Autodesk Fusion 360 part; units mm, degrees
sketch "Sketch1" plane through (0, 0, 0) normal (0, 0, 1) x (1, 0, 0)
  line L0 (0, 0) -> (60, 0)
  line L1 (60, 0) -> (60, 50)
  line L2 (60, 50) -> (0, 50)
  line L3 (0, 50) -> (0, 0)
  line L4 (0, 50) -> (5, 50)
  line L5 (5, 50) -> (5, 47.5)
  line L6 (5, 47.5) -> (0, 47.5)
  line L7 (0, 47.5) -> (0, 50)
  line L8 (0, 0) -> (5, 0)
  line L9 (5, 0) -> (5, 2.5)
  line L10 (5, 2.5) -> (0, 2.5)
  line L11 (0, 2.5) -> (0, 0)
  circle A0 centre (5, 2.5) radius 1.5
  circle A1 centre (5, 47.5) radius 1.5
  line L12 (5, 47.5) -> (35, 47.5)
  line L13 (5, 2.5) -> (35, 2.5)
  line L14 (5, 50) -> (5, 40)
  line L15 (5, 0) -> (5, 10)
  line L16 (5, 40) -> (50, 40)
  line L17 (5, 10) -> (50, 10)
  line L18 (60, 50) -> (60, 45)
  line L19 (60, 45) -> (45, 45)
  circle A2 centre (45, 45) radius 1.25
  line L20 (60, 0) -> (60, 5)
  line L21 (60, 5) -> (45, 5)
  circle A3 centre (45, 5) radius 1.25
  line L22 (60, 0) -> (60, 25)
  line L23 (60, 25) -> (45, 25)
  circle A4 centre (45, 25) radius 6.25
  circle A5 centre (50, 40) radius 1.5
  circle A6 centre (5, 10) radius 1.5
  circle A7 centre (50, 10) radius 1.5
  circle A8 centre (35, 47.5) radius 1.5
  circle A9 centre (35, 2.5) radius 1.5
  dimension "d1" = 60
  dimension "d2" = 50
  dimension "d3" = 5
  dimension "d4" = 2.5
  dimension "d5" = 5
  dimension "d6" = 2.5
  dimension "d7" = 3
  dimension "d8" = 3
  dimension "d9" = 30
  dimension "d10" = 30
  dimension "d11" = 10
  dimension "d12" = 10
  dimension "d13" = 45
  dimension "d14" = 45
  dimension "d15" = 15
  dimension "d16" = 2.5
  dimension "d17" = 5
  dimension "d18" = 15
  dimension "d19" = 2.5
  dimension "d20" = 15
  dimension "d21" = 12.5
  dimension "d22" = 3
  dimension "d23" = 3
  dimension "d24" = 3
  dimension "d25" = 3
  dimension "d26" = 3
extrude "Extrude1" add sketch "Sketch1" along normal blind 5 contours L0 L3 L8 L9 L10 L11 A0 L15 | L0 L1 L2 L3 L5 L6 L9 L10 A0 A1 L14 L15 L18 L20 L22 | L2 L3 L4 L5 L6 L7 A1 L14
sketch "Sketch2" plane through (0, 0, 5) normal (0, 0, 1) x (1, 0, 0)
  circle A0 centre (5, 2.5) radius 1.5
  circle A1 centre (5, 10) radius 1.5
  circle A2 centre (35, 2.5) radius 1.5
  circle A3 centre (45, 45) radius 1.25
  circle A4 centre (35, 47.5) radius 1.5
  circle A5 centre (50, 40) radius 1.5
  circle A6 centre (50, 10) radius 1.5
  circle A7 centre (45, 5) radius 1.25
  circle A8 centre (45, 25) radius 6.25
  circle A9 centre (5, 47.5) radius 1.5
  line L0 (0, 50) -> (0, 0)
  line L1 (0, 0) -> (60, 0)
  line L2 (60, 0) -> (60, 50)
  line L3 (60, 50) -> (0, 50)
  line L4 (50, 40) -> (5, 40)
  circle A10 centre (5, 40) radius 1.5
  dimension "d29" = 45
  dimension "d30" = 3
extrude "Extrude2" cut sketch "Sketch2" against normal blind 5 contours A10
sketch "Sketch3" plane through (0, 0, 0) normal (0, 0, -1) x (-1, 0, 0)
  circle A0 centre (-5, 40) radius 1.5
  circle A1 centre (-5, 2.5) radius 1.5
  circle A2 centre (-5, 10) radius 1.5
  circle A3 centre (-35, 2.5) radius 1.5
  circle A4 centre (-45, 45) radius 1.25
  circle A5 centre (-35, 47.5) radius 1.5
  circle A6 centre (-50, 40) radius 1.5
  circle A7 centre (-50, 10) radius 1.5
  circle A8 centre (-45, 5) radius 1.25
  circle A9 centre (-45, 25) radius 6.25
  circle A10 centre (-5, 47.5) radius 1.5
  line L0 (0, 0) -> (0, 50)
  line L1 (0, 50) -> (-60, 50)
  line L2 (-60, 50) -> (-60, 0)
  line L3 (-60, 0) -> (0, 0)
  line L4 (0, 0) -> (-10, 0)
  line L5 (-10, 0) -> (-14, 0)
  line L6 (-14, 0) -> (-14, 30)
  line L7 (-14, 30) -> (-10, 30)
  line L8 (-10, 30) -> (-10, 0)
  dimension "d33" = 10
  dimension "d34" = 4
  dimension "d35" = 30
extrude "Extrude3" add sketch "Sketch3" along normal blind 20 contours L3 L5 L6 L7 L8
sketch "Sketch4" plane through (0, 0, -20) normal (0, 0, -1) x (-1, 0, 0)
  line L0 (-10, 30) -> (-14, 30)
  line L1 (-14, 30) -> (-14, 0)
  line L2 (-14, 0) -> (-10, 0)
  line L3 (-10, 0) -> (-10, 30)
  line L4 (-14, 30) -> (-10, 30)
  line L5 (-10, 30) -> (-10, 26.5)
  line L6 (-10, 26.5) -> (-14, 26.5)
  line L7 (-14, 26.5) -> (-14, 30)
  line L8 (-10, 0) -> (-14, 0)
  line L9 (-14, 0) -> (-14, 3.5)
  line L10 (-14, 3.5) -> (-10, 3.5)
  line L11 (-10, 3.5) -> (-10, 0)
  dimension "d38" = 3.5
  dimension "d39" = 3.5
extrude "Extrude4" add sketch "Sketch4" along normal blind 10 contours L0 L1 L3 L4 L5 L6 L7 | L1 L2 L3 L8 L9 L10 L11
sketch "Sketch5" plane through (10, 0, 0) normal (-1, 0, 0) x (0, 0, 1)
  line L0 (0, 0) -> (0, 30)
  line L1 (0, 30) -> (-30, 30)
  line L2 (-30, 30) -> (-30, 26.5)
  line L3 (-30, 26.5) -> (-20, 26.5)
  line L4 (-20, 26.5) -> (-20, 3.5)
  line L5 (-20, 3.5) -> (-30, 3.5)
  line L6 (-30, 3.5) -> (-30, 0)
  line L7 (-30, 0) -> (0, 0)
  line L8 (-30, 30) -> (-30, 28.25)
  line L9 (-30, 28.25) -> (-25, 28.25)
  line L10 (-30, 0) -> (-30, 1.75)
  line L11 (-30, 1.75) -> (-25, 1.75)
  circle A0 centre (-25, 28.25) radius 1
  circle A1 centre (-25, 1.75) radius 1
  dimension "d42" = 5
  dimension "d43" = 2
  dimension "d44" = 2
extrude "Extrude5" cut sketch "Sketch5" against normal blind 4 contours A0 | A1
sketch "Sketch6" plane through (0, 0, 0) normal (0, 0, -1) x (-1, 0, 0)
  line L0 (-14, 0) -> (-14, 30)
  line L1 (-14, 30) -> (-10, 30)
  line L2 (-10, 30) -> (-10, 0)
  line L3 (-10, 0) -> (0, 0)
  line L4 (0, 0) -> (0, 50)
  line L5 (0, 50) -> (-60, 50)
  line L6 (-60, 50) -> (-60, 0)
  line L7 (-60, 0) -> (-14, 0)
  circle A0 centre (-5, 47.5) radius 1.5
  circle A1 centre (-45, 25) radius 6.25
  circle A2 centre (-45, 5) radius 1.25
  circle A3 centre (-50, 10) radius 1.5
  circle A4 centre (-50, 40) radius 1.5
  circle A5 centre (-35, 47.5) radius 1.5
  circle A6 centre (-45, 45) radius 1.25
  circle A7 centre (-35, 2.5) radius 1.5
  circle A8 centre (-5, 10) radius 1.5
  circle A9 centre (-5, 2.5) radius 1.5
  circle A10 centre (-5, 40) radius 1.5
  line L8 (-10, 0) -> (-10, 5)
  line L9 (-10, 30) -> (-10, 25)
  line L10 (-10, 5) -> (0, 5)
  line L11 (0, 5) -> (0, 8)
  line L12 (0, 8) -> (-10, 8)
  line L13 (-10, 8) -> (-10, 5)
  line L14 (-10, 25) -> (0, 25)
  line L15 (0, 25) -> (0, 22)
  line L16 (0, 22) -> (-10, 22)
  line L17 (-10, 22) -> (-10, 25)
  dimension "d47" = 5
  dimension "d48" = 3
extrude "Extrude6" add sketch "Sketch6" along normal blind 20 contours L2 L4 L14 L15 L16 L17 | L2 L4 L10 L11 L12 L13
chamfer "Chamfer1" distance 10 distance2 20 2 edges at (0, 23.5, -20) (0, 6.5, -20) measured on face at (12.6667, 12.6667, -20) measured on face at (12.6667, 12.6667, -20)
extrude "Extrude7" add 1 faces at (12.6667, 30, -10) along direction (0, 1, 0) blind 3
extrude "Extrude8" add 1 faces at (24.6667, 0, 3.3333) along direction (0, -1, 0) blind 3
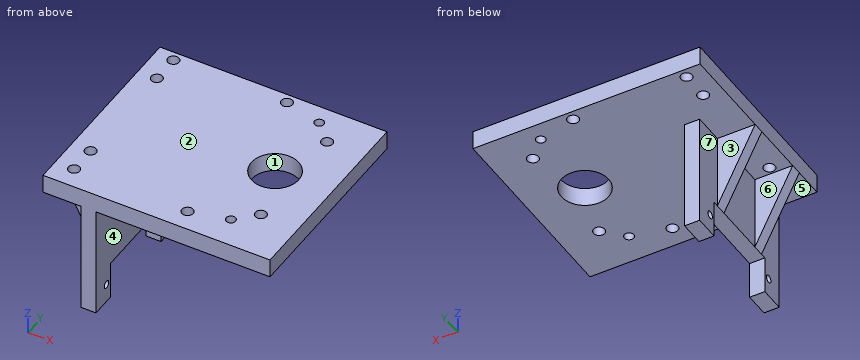
The listing builds one solid part. Answer for the finished solid, in the listing's coordinates (mm). Face numbers are marked on the shaded views. A direction names the side the tool comes from. Give positions to 0.01 mm unless a question says otherwise; leave off trailing zeros. Order: outer loops, then holes, each group sorted by start corner. A loop starts at its lowest first (then second) coordinate and runs counter-clockwise, first axis right, second up. Notation, with made-up numbers: (-34, 52.5) -> (0, 52.5) arc R11 ccw to (0, 73.5) -> close; hole circle Ø11 at (43, 74). An arc over 180 degrees is marked (long way). Answer as a JSON object with one key per item and string values. Group by question number.
Item 1: The part is cut by section D-D on x = 45. Write down the section's boundary in (y, z).
Item 2: The part is cut by section B-B on x = 35. Write down the section's boundary in (y, z).
Item 3: The part is cut by section C-C on z = -25. Write down the section's boundary in (x, y).
Item 4: A tool of negligible diameter and unlimited length cuts with its end or side. For the marked faces 4, 5, 6 and 7, from which of +Z, -Z, +X, -X, +Y, -Y can it reach the whole face along a straight path? Write none if from no direction.
Item 5: The part is cut by section A-A on y = 45. Write down the section's boundary in (x, z), and give its area (4 significant figures).
Item 6: Determine the mould class of the marked faces 1, 2 and 3 for opening direction Y: pulls with the +Y half, pulls with the -Y half, needs draft (parallel to the pull), parting line crosses it, or undercut.
Item 7: Consider L1, parallel to X at y = 40, z = 3; L2, parallel to Y at x = 45, z = 3; L3, parallel to Y at x = 5, z = 3.05. Determine where each line is inside the solid, lowest interval first. Write a range as from..to.
Item 8: Flat-ended cylindrical pins translate along their axes: pin 1 (10 mm diameter, centred on x = 45, y = 25, fed in from +Z); pin 2 (5 mm diameter, centred on x = 50, y = 40, fed in from -Z); pin 3 (5 mm diameter, centred on x = 6.5, z = -11.5, fed in from +Y); pin 4 (5 mm diameter, centred on x = 50, y = 23, fed in from +Z). Find the tip coordinate at first contact, or state that the pin passes through.
Result set:
{
 "1": {"outline": "(-3, 0) -> (3.75, 0) -> (3.75, 5) -> (-3, 5) -> close; (6.25, 0) -> (18.75, 0) -> (18.75, 5) -> (6.25, 5) -> close; (31.25, 0) -> (43.75, 0) -> (43.75, 5) -> (31.25, 5) -> close; (46.25, 0) -> (50, 0) -> (50, 5) -> (46.25, 5) -> close"},
 "2": {"outline": "(-3, 0) -> (1, 0) -> (1, 5) -> (-3, 5) -> close; (4, 0) -> (46, 0) -> (46, 5) -> (4, 5) -> close; (49, 0) -> (50, 0) -> (50, 5) -> (49, 5) -> close"},
 "3": {"outline": "(10, -3) -> (14, -3) -> (14, 0.75) -> (10, 0.75) -> close; (10, 2.75) -> (14, 2.75) -> (14, 3.5) -> (10, 3.5) -> close; (10, 26.5) -> (14, 26.5) -> (14, 27.25) -> (10, 27.25) -> close; (10, 29.25) -> (14, 29.25) -> (14, 33) -> (10, 33) -> close"},
 "4": {"face 4": "-Z, +X, +Y, -Y", "face 5": "-Z, -X, -Y", "face 6": "-Z, -X", "face 7": "-Z, -X, +Y"},
 "5": {"outline": "(0, 0) -> (43.75, 0) -> (43.75, 5) -> (0, 5) -> close; (46.25, 0) -> (60, 0) -> (60, 5) -> (46.25, 5) -> close", "area": "287.5 mm²"},
 "6": {"face 1": "undercut", "face 2": "needs draft", "face 3": "pulls with the +Y half"},
 "7": {"L1": "0..3.5, 6.5..48.5, 51.5..60", "L2": "-3..3.75, 6.25..18.75, 31.25..43.75, 46.25..50", "L3": "-3..1, 4..8.5, 11.5..38.5, 41.5..46, 49..50"},
 "8": {"pin 1": "through", "pin 2": "z = 0", "pin 3": "y = 25", "pin 4": "z = 5"}
}
